```python
from build123d import *

# Parameters (mm, degrees)
F0_W     = 26.5
F0_H     = 94
F1_DEPTH = 6.35
F3_D     = 6.528


with BuildPart() as f1:
    # F0 (on Top) → F1 (new body)
    with BuildSketch(Plane.XY):
        with Locations((0.116214, 19.529511)):
            Rectangle(F0_W, F0_H)
    extrude(amount=F1_DEPTH)

    # F3 (through all)
    with Locations(Plane.XY.offset(6.35)):
        with Locations((0.116214, 61.529511), (0.116214, 41.529511), (0.116214, -22.670489)):
            Hole(F3_D / 2)


solid = f1.part
```
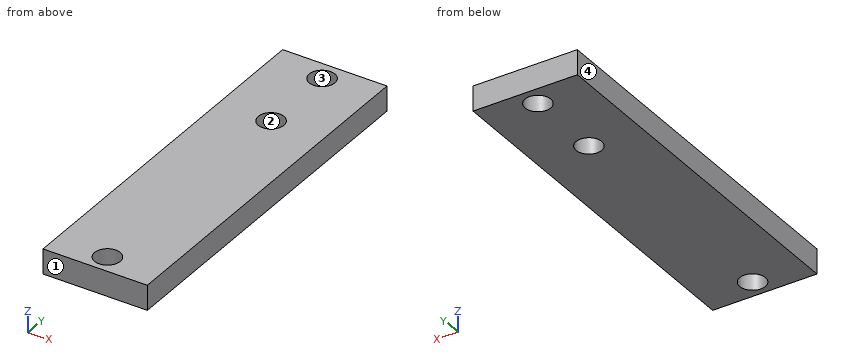
Source: CAD feature listing. Evaluate the final solid. Frame: model axes, mm. Face numbers are marked on the shaded views. Give positions to 0.01 mm unless a question says otherwise; leave off trailing zeros. Order: outer loops, then holes, each group sorted by start corner. A loop starts at its lowest first (then second) coordinate and runs counter-clockwise, first axis right, second up.
(1) Section query A-A (x = 1.25). Return the cut outline in (y, z), plus the area to 3 significant figures.
(2) Material intervals for line 1 along Y through (x, z) = (2, 3); line 2 along Y through (x, z) = (0.25, 2); line 3 along X through (y, z) = (-20, 1.5), sorted ascending.
(3) Section query B-B (z = 4.25). Return the cut outline in (x, y), plus the area to 3 significant figures.
(4) Contact query for a flat-ended pin moving along its axis: P1, Ø5, axis at x = 0.12, y = 61.53, coming from the -Z side (1 decimal). Output: stop coordinate, or through.
(5) Pull-direction query (Y, two-part tool) for the marked faces 1, 2, 3 and 4; classes: +Y half, -Y half, draft (parallel to the pull), parting line (faces both ways), or undercut.
Outcome:
1. outline: (-27.47, 0) - (-25.73, 0) - (-25.73, 6.35) - (-27.47, 6.35) - close; (-19.61, 0) - (38.47, 0) - (38.47, 6.35) - (-19.61, 6.35) - close; (44.59, 0) - (58.47, 0) - (58.47, 6.35) - (44.59, 6.35) - close; (64.59, 0) - (66.53, 0) - (66.53, 6.35) - (64.59, 6.35) - close
1. area: 480 mm2
2. line 1: y = -27.47 to -25.34, -20 to 38.86, 44.2 to 58.86, 64.2 to 66.53
2. line 2: y = -27.47 to -25.93, -19.41 to 38.27, 44.79 to 58.27, 64.79 to 66.53
2. line 3: x = -13.13 to -1.76, 1.99 to 13.37
3. outline: (-13.13, -27.47) - (13.37, -27.47) - (13.37, 66.53) - (-13.13, 66.53) - close; hole circle Ø6.53 at (0.12, -22.67); hole circle Ø6.53 at (0.12, 41.53); hole circle Ø6.53 at (0.12, 61.53)
3. area: 2,390 mm2
4. P1: passes through
5. face 1: -Y half
5. face 2: undercut
5. face 3: undercut
5. face 4: draft
